For this review, take the finished solid that the model builds, in its own axes (mm). A direction names the side the tool comes from. Give positions to 0.01 mm unless a question says otherwise; leave off trailing zeros. Order: outer loops, then holes, each group sorted by start corner. A loop starts at its lowest first (then second) coordinate and runs counter-clockwise, first axis right, second up. Notation, with made-up numbers: M 9,-11.75 L 21,-11.75 A13 cw 21,0.25 Z; hole C 1.5,74.25 d6. An arc over 180 degrees is marked long. Use CSV: the item, a comma, the result in double quotes. Start each with the question number.
(1) Wall thickness on L1, parallel to Y at x = 10, z = 0.4; L2, parallel to Y at x = -4, z = 0; L3, parallel to Y at x = -20, z = -0.15: over which ranges is each line inside the solid? List them lowest first. Write a range as from..to.
(2) Tool access review of faces 4 (the face through (13.13, 43.36, 0.01)), 5 (the face through (11, 19.05, 0)), 6 (the face through (-4, 31.75, 0)): name each direction out of +Z, -Z, +X, -X, +Y, -Y from which nothing blocks a thin tool from reaching the whole face with its end or side.
(3) Consider section A-A (y = 50.8). Write out the cut boundary in (x, z).
(4) Draft analysis for pull direction X (two halves, no side actions). For faces 1 (the face through (2.435, 0.767, -0.008)), 2 (the face through (-14, 6.35, 0)), 3 (the face through (-14.71, 46.04, 0.01)), state which applies: pulls with the +X half, pulls with the -X half, needs draft (parallel to the pull), parting line crosses it, or undercut.
(5) Clearance check with a flat-ended pin moving along its axis: P1, Ø0.6, axis at x = -3.5, z = 0, coming from the -Y side. State where the tip first meets the part, or that it passes through.
(6) Consider section B-B (z = -0.1). Give the number of separate pieces and of enclosed holes in the cut face, and give its area (3 significant figures).
(7) Consider section C-C (y = 43.5). Write out the cut boundary in (x, z), and give its area (3 significant figures).
```python
from build123d import *

# Parameters (mm, degrees)
SKETCH1_R           = 2.5527
SKETCH1_W           = 7.9248
SKETCH1_H           = 12.7
BOSS_EXTRUDE1_DEPTH = 0.5842
FILLET1_R           = 3.81
FILLET2_R           = 1.524


with BuildPart() as part:
    # Sketch1 → Boss-Extrude1 (new body, symmetric)
    with BuildSketch(Plane.XY):
        with BuildLine():
            ThreePointArc((-4.612542275, 1.419411765), (0, -4.826), (4.612542275, 1.419411765))
            ThreePointArc((4.612542275, 1.419411765), (5.18926029, 4.803477283), (8.254023019, 6.35))
            Line((8.254023019, 6.35), (14.2748, 6.35))
            Line((14.2748, 6.35), (14.2748, 19.05))
            Line((14.2748, 19.05), (6.35, 19.05))
            Line((6.35, 19.05), (6.35, 31.75))
            Line((6.35, 31.75), (14.2748, 31.75))
            Line((14.2748, 31.75), (14.2748, 44.45))
            Line((14.2748, 44.45), (-1.296376981, 44.45))
            ThreePointArc((-1.296376981, 44.45), (-4.36113971, 45.996522717), (-4.937857725, 49.380588235))
            ThreePointArc((-4.937857725, 49.380588235), (-9.5504, 55.626), (-14.162942275, 49.380588235))
            ThreePointArc((-14.162942275, 49.380588235), (-14.73966029, 45.996522717), (-17.804423019, 44.45))
            Line((-17.804423019, 44.45), (-23.8252, 44.45))
            Line((-23.8252, 44.45), (-23.8252, 6.35))
            Line((-23.8252, 6.35), (-8.254023019, 6.35))
            ThreePointArc((-8.254023019, 6.35), (-5.18926029, 4.803477283), (-4.612542275, 1.419411765))
        make_face()
        Circle(SKETCH1_R, mode=Mode.SUBTRACT)
        with Locations((-9.5504, 50.8)):
            Circle(SKETCH1_R, mode=Mode.SUBTRACT)
        with Locations((-3.9624, 25.4)):
            Rectangle(SKETCH1_W, SKETCH1_H, mode=Mode.SUBTRACT)
    extrude(amount=BOSS_EXTRUDE1_DEPTH, both=True)

    # Fillet1
    fillet1_edges = [part.edges().sort_by_distance(p)[0] for p in [
        (-23.8252, 6.35, 0),
        (-23.8252, 44.45, 0),
        (14.2748, 44.45, 0),
        (14.2748, 6.35, 0),
    ]]
    fillet(fillet1_edges, radius=FILLET1_R)

    # Fillet2
    fillet2_edges = [part.edges().sort_by_distance(p)[0] for p in [
        (6.35, 31.75, 0),
        (6.35, 19.05, 0),
        (-7.9248, 19.05, 0),
        (0, 19.05, 0),
        (0, 31.75, 0),
        (-7.9248, 31.75, 0),
    ]]
    fillet(fillet2_edges, radius=FILLET2_R)


solid = part.part
```
Check result:
1,L1,"y = 6.35..19.05, 31.75..44.45"
1,L2,"y = -2.7..19.05, 31.75..45.58"
1,L3,"y = 6.35..44.45"
2,face 4,"+Z, -Z, +X, +Y"
2,face 5,"+Z, -Z, +X"
2,face 6,"+Z, -Z"
3,outline,"M -14.38,-0.58 L -12.1,-0.58 L -12.1,0.58 L -14.38,0.58 Z; M -7,-0.58 L -4.72,-0.58 L -4.72,0.58 L -7,0.58 Z"
4,face 1,"undercut"
4,face 2,"needs draft"
4,face 3,"pulls with the -X half"
5,P1,"stops at y = -3.61"
6,separate pieces,"1"
6,enclosed holes,"3"
6,area,"1,400 mm^2"
7,outline,"M -22.53,-0.58 L 12.98,-0.58 L 12.98,0.58 L -22.53,0.58 Z"
7,area,"41.5 mm^2"
